Verification items for the finished model (mm, model axes). A direction names the side the tool comes from. Coordinates: 2 decimals unless noted, no trailing zeros. Order: outer loops, then holes, each group sorted by start corner. A loop starts at its lowest first (then second) coordinate and runs counter-clockwise, first axis right, second up. Notation, with made-up numbers: (5, 88.25) -> (17, 88.25) arc R8 cw to (17, 94.25) -> close; hole circle Ø11 at (19.25, 21.5). An arc over 180 degrees is marked (long way). Write item = value, one per line. Start each with the question number.
from build123d import *

# Parameters (mm, degrees)
F0_R     = 10
F1_DEPTH = 150
F0_R_2   = 30
F2_DEPTH = 80
F0_R_3   = 50
F3_DEPTH = 40


with BuildPart() as f1:
    # F0 (on Front) → F1 (new body)
    with BuildSketch(Plane.XZ):
        Circle(F0_R)
    extrude(amount=F1_DEPTH)

    # F0 (on Front) → F2 (join)
    with BuildSketch(Plane.XZ):
        Circle(F0_R_2)
        Circle(F0_R, mode=Mode.SUBTRACT)
    extrude(amount=F2_DEPTH)

    # F0 (on Front) → F3 (join)
    with BuildSketch(Plane.XZ):
        Circle(F0_R_3)
        Circle(F0_R_2, mode=Mode.SUBTRACT)
    extrude(amount=F3_DEPTH)

    # F4: F1 across plane


with BuildPart() as f1_1:
    add(f1.part)
    add(f1.part.mirror(Plane.XZ))


solid = f1_1.part
Item 1: Section check B-B (x = 0). Record the boundary of the cut face in (y, z).
Item 2: Tool access check on faces 1 (the cylindrical face through (-2.17, 114.51, -9.76)), 2 (the cylindrical face through (-2.17, -114.51, -9.76)), 3 (the cylindrical face through (47.69, -0.56, 15.02)). Record the directions out of +Z, -Z, +X, -X, +Y, -Y that give a thin tool (end or side, any length) a straight path to the whole face; none if there is none.
Item 3: Gauge pin test, flat ends, axial feed: P1, Ø10, axis at x = 21, y = -1.5, coming from the +Z side; P2, Ø6, axis at x = -38.5, z = -38, coming from the +Y side; P3, Ø8, axis at x = -14, z = 5.5, coming from the -Y side; P4, Ø10, axis at x = -4.5, y = -118.5, coming from the -Z side. Record the tip position at first contact, or that the pin passes through.
Item 4: Thickness scan on line 1 (Y direction, x = -3, z = 38); line 2 (Y direction, x = -24, z = 1.5); line 3 (Z direction, x = -40, y = -10). Record the ranges inside material, lowest first.
Item 5: Section check C-C (y = 9). Record the boundary of the cut face in (x, z).
Item 6: Section check A-A (z = 0). Record the boundary of the cut face in (x, y).
Item 7: Mould release check, pull along X, two halves, no side actions. Record for faces 4 (the cylindrical face through (-29.97, -59.72, 1.32)), 5 (the flat face through (22, 40, -22)): pulls with the +X half, pulls with the -X half, needs draft (parallel to the pull), parting line crosses it, or undercut.
Item 8: Section check D-D (x = 18). Record the boundary of the cut face in (y, z).
Filled sheet:
q1.outline = (-150, -10) -> (-80, -10) -> (-80, -30) -> (-40, -30) -> (-40, -50) -> (40, -50) -> (40, -30) -> (80, -30) -> (80, -10) -> (150, -10) -> (150, 10) -> (80, 10) -> (80, 30) -> (40, 30) -> (40, 50) -> (-40, 50) -> (-40, 30) -> (-80, 30) -> (-80, 10) -> (-150, 10) -> close
q2.face_1 = +Y
q2.face_2 = -Y
q2.face_3 = +Y, -Y
q3.P1 = 47.37
q3.P2 = through
q3.P3 = -80
q3.P4 = -10
q4.line_1 = -40 to 40
q4.line_2 = -80 to 80
q4.line_3 = -30 to 30
q5.outline = circle Ø100 at (0, 0)
q6.outline = (-50, -40) -> (-30, -40) -> (-30, -80) -> (-10, -80) -> (-10, -150) -> (10, -150) -> (10, -80) -> (30, -80) -> (30, -40) -> (50, -40) -> (50, 40) -> (30, 40) -> (30, 80) -> (10, 80) -> (10, 150) -> (-10, 150) -> (-10, 80) -> (-30, 80) -> (-30, 40) -> (-50, 40) -> close
q7.face_4 = parting line crosses it
q7.face_5 = needs draft
q8.outline = (-80, -24) -> (-40, -24) -> (-40, -46.65) -> (40, -46.65) -> (40, -24) -> (80, -24) -> (80, 24) -> (40, 24) -> (40, 46.65) -> (-40, 46.65) -> (-40, 24) -> (-80, 24) -> close
